from build123d import *

# Parameters (mm, degrees)
F2_R = 0.8


with BuildPart() as f1:
    # F0 (on Front) → F1 (revolve)
    with BuildSketch(Plane.XZ):
        Polygon((2.2, 0), (5, 0), (5, 0.8), (3, 0.8), (2.15, 10), (0, 10), (0, 9.2), (1.35, 9.2), align=None)
    revolve(axis=Axis((0, 0, 4.745889), (0, 0, -1)))

    # F2
    f2_edges = [f1.edges().sort_by_distance(p)[0] for p in [
        (-2.15, 0, 10),
    ]]
    fillet(f2_edges, radius=F2_R)


solid = f1.part
Could you check a few things on this model? Use its own coordinates, in mm. Give positions to 0.01 mm unless a question says otherwise; leave off trailing zeros. Loops run counter-clockwise (first coordinate to the right, second up) from the corner with the lowest first, then second, coordinate; pieces in that order, holes last. Notation, with made-up numbers: (36, 39) -> (74, 39) arc R18 ccw to (74, 58) -> close; hole circle Ø4 at (-9, -35). An arc over 180 degrees is marked (long way). Return JSON: item names as keys, results as strings.
Item 1: We'd pull the mould along X, two halves only. Please class faces 1 (the flat face through (0, 0, 9.2)), 2 (the flat face through (3.3, -0.1, 0.8)), 3 (the conical face through (2.483, -0.782, 5.096)): +X half, -X half, draft (parallel to the pull), parting line (faces both ways), or undercut.
Geometry results:
{"face 1": "undercut", "face 2": "draft", "face 3": "parting line"}
Item 2: I'm going to push flat-ended pins straight in: pin 1 (2 mm diameter, centred on x = 0, y = 0, fed in from -Z); pin 2 (3 mm diameter, centred on y = 2.5, z = 4, fed in from -X); pin 3 (3 mm diameter, centred on x = -3.5, z = 6, fed in from +Y); pin 4 (4 mm diameter, centred on x = 0.5, y = -4, fed in from -Z). Where does each tip first touch, or does it pass through?
Geometry results:
{"pin 1": "stops at z = 9.2", "pin 2": "stops at x = -2.53", "pin 3": "stops at y = 1.55", "pin 4": "stops at z = 0"}
Item 3: If we section it at D-D on z = 5.75: List the corners of the cut face in (x, y) for me.
Geometry results:
{"outline": "circle Ø5.09 at (0, 0); hole circle Ø3.34 at (0, 0)"}
Item 4: If we section it at C-C on z = 9: List the corners of the cut face in (x, y) for me.
Geometry results:
{"outline": "circle Ø4.48 at (0, 0); hole circle Ø2.74 at (0, 0)"}
Item 5: I need wall thicknesses on L1, parallel to Z at x = -2.25, y = 3.5; L2, parallel to X at y = -0.25, z = 2.5; L3, parallel to Y at x = -0.5, z = 2.5. Which ranges of each line are inside material? Lowest first, please. Write a range as from..to.
Geometry results:
{"L1": "z = 0..0.8", "L2": "x = -2.83..-1.95, 1.95..2.83", "L3": "y = -2.8..-1.9, 1.9..2.8"}
Item 6: If we section it at A-A on x = 0: List the corners of the cut face in (y, z) for me.
Geometry results:
{"outline": "(-5, 0) -> (-2.2, 0) -> (-1.35, 9.2) -> (1.35, 9.2) -> (2.2, 0) -> (5, 0) -> (5, 0.8) -> (3, 0.8) -> (2.22, 9.27) arc R0.8 ccw to (1.42, 10) -> (-1.42, 10) arc R0.8 ccw to (-2.22, 9.27) -> (-3, 0.8) -> (-5, 0.8) -> close"}
